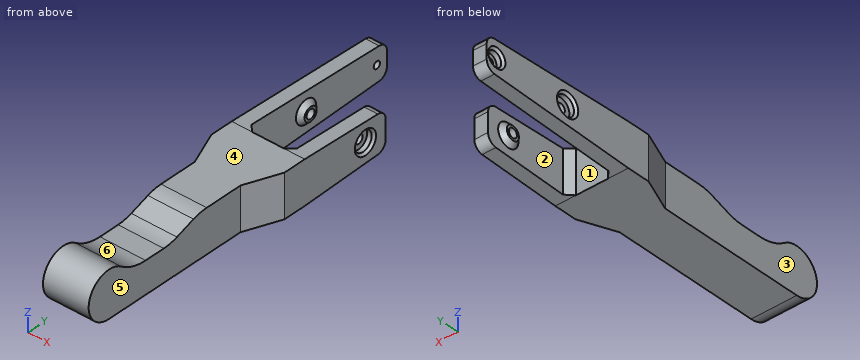
```python
from build123d import *

# Parameters (mm, degrees)
SKETCH1_R           = 2
BOSS_EXTRUDE1_DEPTH = 6
SKETCH2_R           = 4.25
CUT_EXTRUDE1_DEPTH  = 3
SKETCH3_W           = 18.888907728
SKETCH3_H           = 10
BOSS_EXTRUDE2_DEPTH = 32
BOSS_EXTRUDE3_START = -6
SKETCH4_R           = 2
BOSS_EXTRUDE3_DEPTH = 6
FILLET1_R           = 4
CUT_EXTRUDE2_START  = -29
SKETCH2_2_R         = 4.25
CUT_EXTRUDE2_DEPTH  = 3
CHAMFER1_SIZE       = 1
CHAMFER2_SIZE       = 3
SKETCH5_R           = 3
SKETCH5_R_2         = 2
BOSS_EXTRUDE4_DEPTH = 2
BOSS_EXTRUDE5_START = 18
SKETCH5_2_R         = 3
SKETCH5_2_R_2       = 2
BOSS_EXTRUDE5_DEPTH = 2
CHAMFER4_SIZE       = 2
BOSS_EXTRUDE6_DEPTH = 18.888907729
BOSS_EXTRUDE7_DEPTH = 20
CHAMFER5_SIZE       = 15
CHAMFER5_SIZE_2     = 5.164914199
FILLET2_R           = 20
SKETCH9_R           = 1.55
CUT_EXTRUDE3_DEPTH  = 6
CUT_EXTRUDE4_START  = -3
SKETCH10_R          = 3.25
SKETCH10_R_2        = 1.55
CUT_EXTRUDE4_DEPTH  = 3
CHAMFER6_SIZE       = 1


# Some blends are built 0.0001 mm under size
with BuildPart() as part:
    # Sketch1 → Boss-Extrude1 (new body)
    with BuildSketch(Plane(origin=(0, 0, 0), x_dir=(0, 0, -1), z_dir=(1, 0, 0))):
        Polygon((-9.444453864, -30), (-7, 40), (7, 40), (9.444453864, -30), align=None)
        Circle(SKETCH1_R, mode=Mode.SUBTRACT)
    extrude(amount=BOSS_EXTRUDE1_DEPTH)

    # Sketch2 → Cut-Extrude1 (cut)
    with BuildSketch(Plane.ZY):
        Circle(SKETCH2_R)
    extrude(amount=-CUT_EXTRUDE1_DEPTH, mode=Mode.SUBTRACT)

    # Sketch3 → Boss-Extrude2 (add)
    with BuildSketch(Plane.ZY):
        with Locations((0, -35)):
            Rectangle(SKETCH3_W, SKETCH3_H)
    extrude(amount=-BOSS_EXTRUDE2_DEPTH)

    # Sketch4 → Boss-Extrude3 (add)
    with BuildSketch(Plane(origin=(32, 0, 0), x_dir=(0, 0, -1), z_dir=(1, 0, 0)).offset(BOSS_EXTRUDE3_START)):
        Polygon((9.444453864, -30), (-9.444453864, -30), (-8.047623085, 10), (8.047623085, 10), align=None)
        with Locations(Location((0, 0, 0), (0, 0, 180))):
            Circle(SKETCH4_R, mode=Mode.SUBTRACT)
    extrude(amount=BOSS_EXTRUDE3_DEPTH)

    # Fillet1
    fillet1_edges = [part.edges().sort_by_distance(p)[0] for p in [
        (29, 10, -8.047623085),
        (29, 10, 8.047623085),
        (3, 40, 7),
        (3, 40, -7),
    ]]
    fillet(fillet1_edges, radius=FILLET1_R)

    # Sketch2<2> → Cut-Extrude2 (cut)
    with BuildSketch(Plane.ZY.offset(CUT_EXTRUDE2_START)):
        Circle(SKETCH2_2_R)
    extrude(amount=-CUT_EXTRUDE2_DEPTH, mode=Mode.SUBTRACT)

    # Chamfer1
    chamfer1_edges = [part.edges().sort_by_distance(p)[0] for p in [
        (0, 0, -4.25),
        (32, 0, -4.25),
    ]]
    chamfer(chamfer1_edges, length=CHAMFER1_SIZE)

    # Chamfer2
    chamfer2_edges = [part.edges().sort_by_distance(p)[0] for p in [
        (26, -30, 0),
        (6, -30, 0),
    ]]
    chamfer(chamfer2_edges, length=CHAMFER2_SIZE)

    # Sketch5 → Boss-Extrude4 (add)
    with BuildSketch(Plane(origin=(6, 0, 0), x_dir=(0, 0, -1), z_dir=(1, 0, 0))):
        with Locations(Location((0, 0, 0), (0, 0, 180))):
            Circle(SKETCH5_R)
        with Locations(Location((0, 0, 0), (0, 0, 180))):
            Circle(SKETCH5_R_2, mode=Mode.SUBTRACT)
    extrude(amount=BOSS_EXTRUDE4_DEPTH)

    # Sketch5<2> → Boss-Extrude5 (add)
    with BuildSketch(Plane(origin=(6, 0, 0), x_dir=(0, 0, -1), z_dir=(1, 0, 0)).offset(BOSS_EXTRUDE5_START)):
        with Locations(Location((0, 0, 0), (0, 0, 180))):
            Circle(SKETCH5_2_R)
        with Locations(Location((0, 0, 0), (0, 0, 180))):
            Circle(SKETCH5_2_R_2, mode=Mode.SUBTRACT)
    extrude(amount=BOSS_EXTRUDE5_DEPTH)

    # Chamfer4
    chamfer4_edges = [part.edges().sort_by_distance(p)[0] for p in [
        (6, 0, -3),
        (26, 0, -3),
    ]]
    chamfer(chamfer4_edges, length=CHAMFER4_SIZE - 0.0001)  # a hair under: the kernel refuses the full size

    # Sketch7 → Boss-Extrude6 (add)
    with BuildSketch(Plane(origin=(0, 0, -9.444453864), x_dir=(-1, 0, 0), z_dir=(0, 0, -1))):
        Polygon((-32, -40), (-26, -55), (-26, -60), (-6, -60), (-6, -55), (0, -40), align=None)
    extrude(amount=-BOSS_EXTRUDE6_DEPTH)

    # Sketch8 → Boss-Extrude7 (add)
    with BuildSketch(Plane(origin=(26, 0, 0), x_dir=(0, 0, -1), z_dir=(1, 0, 0))):
        with BuildLine():
            Line((9.444453864, -60), (-9.444453864, -60))
            Line((-9.444453864, -60), (-9.444453864, -90))
            Line((-9.444453864, -90), (-4.444453864, -90))
            Line((-4.444453864, -90), (-4.444453864, -110.787161313))
            ThreePointArc((-4.444453864, -110.787161313), (-6.083245599, -128.333338985), (9.444453864, -120))
            Line((9.444453864, -120), (9.444453864, -60))
        make_face()
    extrude(amount=-BOSS_EXTRUDE7_DEPTH)

    # Chamfer5
    # the kernel refuses this chamfer: 15, 5.164914199 mm, written as the material it takes off along each edge
    with BuildSketch(Plane(origin=(64.9213417, -90, 9.444453864), x_dir=(0, 0.9999212813122312, 0.012547158200392249), z_dir=(-1, 0, 0))) as chamfer5_piece_1_section:
        Polygon((CHAMFER5_SIZE * 0.999921281312, CHAMFER5_SIZE * 0.0125471582004), (-CHAMFER5_SIZE_2 * 0.0125471582012, CHAMFER5_SIZE_2 * 0.999921281379), (0, 0), align=None)
    chamfer5_piece_1 = extrude(amount=97.842683401, mode=Mode.PRIVATE)
    chamfer5_piece_1 = split(chamfer5_piece_1, bisect_by=Plane(origin=(16, -84.819367326, 4.444453864), z_dir=(0, 0, 1)), keep=Keep.TOP, mode=Mode.PRIVATE)
    add(chamfer5_piece_1, mode=Mode.SUBTRACT)

    # Fillet2
    fillet2_edges = [part.edges().sort_by_distance(p)[0] for p in [
        (16, -110.787161313, 4.444453864),
        (16, -75, 9.444453864),
        (16, -89.521054388, 4.444453864),
    ]]
    fillet(fillet2_edges, radius=FILLET2_R)

    # Sketch9 → Cut-Extrude3 (cut)
    with BuildSketch(Plane(origin=(6, 0, 0), x_dir=(0, 0, -1), z_dir=(1, 0, 0))):
        with Locations((0, 35)):
            Circle(SKETCH9_R)
    extrude(amount=-CUT_EXTRUDE3_DEPTH, mode=Mode.SUBTRACT)

    # Sketch10 → Cut-Extrude4 (cut)
    with BuildSketch(Plane.ZY.offset(CUT_EXTRUDE4_START)):
        with Locations((0, 35)):
            Circle(SKETCH10_R)
        with Locations(Location((0, 35, 0), (0, 0, 180))):
            Circle(SKETCH10_R_2, mode=Mode.SUBTRACT)
    extrude(amount=CUT_EXTRUDE4_DEPTH, mode=Mode.SUBTRACT)

    # Chamfer6
    chamfer6_edges = [part.edges().sort_by_distance(p)[0] for p in [
        (0, 35, -3.25),
    ]]
    chamfer(chamfer6_edges, length=CHAMFER6_SIZE)


solid = part.part
```
The model under review builds one solid part; all positions refer to its coordinate system, in mm. Face numbers are marked on the shaded views. A direction names the side the tool comes from. Give positions to 0.01 mm unless a question says otherwise; leave off trailing zeros. Write each loop counter-clockwise with the first axis right and the second up, starting at its lowest first coordinate (ties: lowest second). Pieces come first, ordered by that corner, then holes. Notation, with made-up numbers: M 34.5,55 L 38.5,55 A18 ccw 38.5,86 Z; hole C -37,63.5 d8. An arc over 180 degrees is marked long. Write each question's results on one line, items separated by ' | '. Start each with the question number.
1. We need section A-A (x = 18.5). Write out the cut boundary in (y, z).
2. We need section D-D (y = -118). Write out the cut boundary in (x, z).
3. Mouldability with a two-part tool opening along Y and no side actions: class the marked faces 1, 2 and 3 as released by +Y, released by -Y, zero draft, split by the parting line, or undercut.
4. We need section B-B (y = -96). Write out the cut boundary in (x, z), and give its area (3 significant figures).
5. Insertion check: pin 1 Ø4 at (y, z) = (-99, 1.5) entering from -X; pin 2 Ø10 at (y, z) = (-89, -3) entering from +X; pin 3 Ø4 at (x, y) = (21, -47) entering from +Z. Each pin has a flat end and moves straight along its axis. Give the tip position at first contact, or say it passes through.
6. For probe 1 along X at (y, z) = (-26, 3.5); probe 2 along X at (y, z) = (-106, -0.5); probe 3 along X at (y, z) = (11.5, 4.25), list the stretches that pass through material, from the lowest coordinate up. Write a range as [from, to].
7. For the marked faces 4, 5 and 6, list the 3-axis set-ups (+Z, -Z, +X, -X, +Y, -Y) from which the entire face can be reached by the end or side of a thin tool; tool diameter is ignored.
Results found:
1) outline: M -120,-9.44 L -30,-9.44 L -30,9.44 L -71.65,9.44 A20 ccw -78.16,8.35 L -86.36,5.53 A20 cw -92.87,4.44 L -101.85,4.44 A20 cw -113.95,8.52 A10 ccw long Z
2) outline: M 6,-9.44 L 26,-9.44 L 26,10.35 L 6,10.35 Z
3) face 1: released by +Y | face 2: undercut | face 3: zero draft
4) outline: M 6,-9.44 L 26,-9.44 L 26,4.44 L 6,4.44 Z | area: 278 mm^2
5) pin 1: stops at x = 6 | pin 2: stops at x = 26 | pin 3: stops at z = 9.44
6) probe 1: x = [0, 6], [26, 32] | probe 2: x = [6, 26] | probe 3: x = [0, 6]
7) face 4: +Z, +X, -X, +Y | face 5: +Z, -Z, +X, -Y | face 6: +Z, +X, -X
